Verification items for the finished model (mm, model axes). Round coordinates to 2 decimals unless told otherwise and drop trailing zeros. Write each loop counter-clockwise with the first axis right and the second up, starting at its lowest first coordinate (ties: lowest second). Pieces come first, ordered by that corner, then holes. Notation, with made-up numbers: (4, 68.5) - (29, 68.5) arc R20 cw to (29, 100.5) - close; hole circle Ø5 at (-19.75, 36). An arc over 180 degrees is marked (long way). Answer as a JSON object with one key per item and string values.
```python
from build123d import *

# Parameters (mm, degrees)
F0_W     = 152.4
F0_H     = 152.4
F1_DEPTH = 1.5875
F2_R     = 7.62
F3_W     = 101.6
F3_H     = 101.6
F4_DEPTH = 1.5885


with BuildPart() as f1:
    # F0 (on Top) → F1 (new body)
    with BuildSketch(Plane.XY):
        Rectangle(F0_W, F0_H)
    extrude(amount=F1_DEPTH)

    # F2
    f2_edges = [f1.edges().sort_by_distance(p)[0] for p in [
        (76.2, 76.2, 0.79375),
        (-76.2, -76.2, 0.79375),
        (76.2, -76.2, 0.79375),
        (-76.2, 76.2, 0.79375),
    ]]
    fillet(f2_edges, radius=F2_R)

    # F3 (on face) → F4 (cut, through all)
    with BuildSketch(Plane.XY.offset(1.5875)):
        Rectangle(F3_W, F3_H)
    extrude(amount=-F4_DEPTH, mode=Mode.SUBTRACT)


solid = f1.part
```
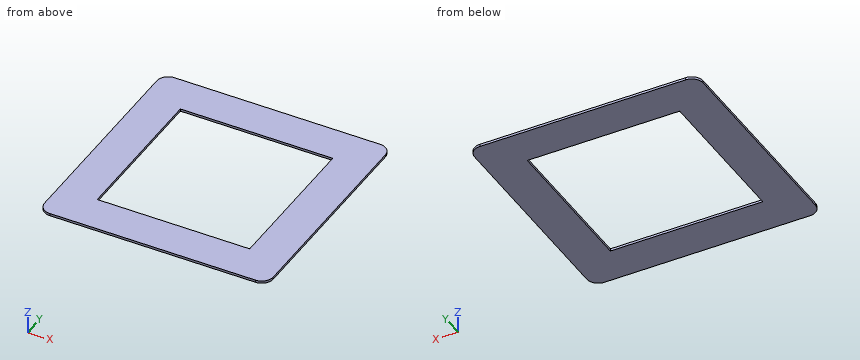
1. Cross-section at A-A (y = 46). Record the boundary of the cut face in (x, z).
Completed:
{"outline": "(-76.2, 0) - (-50.8, 0) - (-50.8, 1.59) - (-76.2, 1.59) - close; (50.8, 0) - (76.2, 0) - (76.2, 1.59) - (50.8, 1.59) - close"}
2. Material ranges on probe 1 along X at (y, z) = (-50, 0.25), recorded low to high. Write a range as from..to.
Completed:
{"probe 1": "x = -76.2..-50.8, 50.8..76.2"}
3. Cross-section at C-C (z = 1.05). Record the boundary of the cut face in (x, y), plus the area to 3 significant figures.
Completed:
{"outline": "(-76.2, -68.58) arc R7.62 ccw to (-68.58, -76.2) - (68.58, -76.2) arc R7.62 ccw to (76.2, -68.58) - (76.2, 68.58) arc R7.62 ccw to (68.58, 76.2) - (-68.58, 76.2) arc R7.62 ccw to (-76.2, 68.58) - close; hole (-50.8, -50.8) - (50.8, -50.8) - (50.8, 50.8) - (-50.8, 50.8) - close", "area": "12,900 mm^2"}
